Geometry: final body of the model. Coordinates: model frame, mm. Face numbers are marked on the shaded views. A direction names the side the tool comes from. Coordinates: 2 decimals unless noted, no trailing zeros. Order: outer loops, then holes, each group sorted by start corner. A loop starts at its lowest first (then second) coordinate and runs counter-clockwise, first axis right, second up. Notation, with made-up numbers: M 8,9.5 L 42,9.5 A8 cw 42,16.5 Z; hole C 70,74.5 d1. An arc over 180 degrees is marked long. Use CSV: the item, a comma, the result in double quotes. Start each with the question number.
1. Section query D-D on x = 40. Return the cut outline in (y, z), and give its area (3 significant figures).
2. Set-up query: the marked faces 4 and 5. Return all of +Z, -Z, +X, -X, +Y, -Y with unobstructed straight access to the full face (end or side cutting, diameter ignored); none if empty.
3. Pull-direction query (Y, two-part tool) for the marked faces 1, 2 and 3; classes: pulls with the +Y half, pulls with the -Y half, needs draft (parallel to the pull), parting line crosses it, or undercut.
4. First-contact query: P1, Ø4.5, axis at x = -15.5, y = -15.5, coming from the -Z side; P2, Ø2, axis at x = -17, y = 11, coming from the +Z side; P3, Ø12, axis at x = -18, z = 2.5, coming from the -Y side. Flat tips, straight axial feed; report the tip coordinate or a pass-through.
5. Section query A-A on y = 0. Return the cut outline in (x, z).
6. Section query B-B on z = 8.5. Return the cut outline in (x, y), and give its area (3 significant figures).
7. Material intervals for line 1 (Y direction, x = -15.5, z = 2.9); line 2 (Y direction, x = -15.5, z = 9.75), sorted ascending.
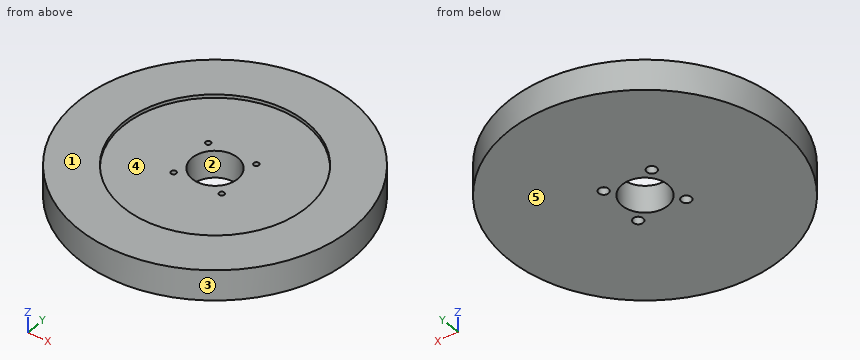
Autodesk Fusion 360 part; units mm, degrees
sketch "Sketch1" plane through (0, 0, 0) normal (0, 0, 1) x (1, 0, 0)
  circle A0 centre (0, 0) radius 90
  circle A1 centre (0, 0) radius 15
  line L0 (15.5, 15.5) -> (-15.5, 15.5)
  line L1 (-15.5, 15.5) -> (-15.5, -15.5)
  line L2 (-15.5, -15.5) -> (15.5, -15.5)
  line L3 (15.5, -15.5) -> (15.5, 15.5)
  line L4 (15.5, 15.5) -> (-15.5, -15.5) construction
  line L5 (-15.5, 15.5) -> (15.5, -15.5) construction
  circle A2 centre (-15.5, 15.5) radius 1.7
  circle A3 centre (15.5, 15.5) radius 1.7
  circle A4 centre (-15.5, -15.5) radius 1.7
  circle A5 centre (15.5, -15.5) radius 1.7
  dimension "d1" = 180
  dimension "d2" = 30
  dimension "d3" = 31
  dimension "d4" = 31
  dimension "d5" = 3.4
  dimension "d8" = 31
  dimension "d9" = -31
extrude "Extrude1" add sketch "Sketch1" along normal blind 20 contours A0 | L0 L1 L2 L3 A2 A3 A4 A5
sketch "Sketch2" plane through (0, 0, 20) normal (0, 0, 1) x (-1, 0, 0)
  circle A0 centre (0, 0) radius 15
  circle A1 centre (15.5, -15.5) radius 1.7
  circle A2 centre (15.5, 15.5) radius 1.7
  circle A3 centre (-15.5, -15.5) radius 1.7
  circle A4 centre (-15.5, 15.5) radius 1.7
  circle A5 centre (0, 0) radius 90
  circle A6 centre (0, 0) radius 60.25
  dimension "d12" = 120.5
extrude "Extrude2" cut sketch "Sketch2" against normal blind 2.2 contours A6
hole "Hole1" at (15.5, -15.5, 0) direction (0, 0, 1) diameter 3.2 depth 17.8 tip angle 118 counterbore diameter 6.5 counterbore depth 5
hole "Hole2" at (15.5, 15.5, 0) direction (0, 0, 1) diameter 3.2 depth 17.8 tip angle 118 counterbore diameter 6.5 counterbore depth 5
hole "Hole3" at (-15.5, -15.5, 0) direction (0, 0, 1) diameter 3.2 depth 17.8 tip angle 118 counterbore diameter 6.5 counterbore depth 5
hole "Hole4" at (-15.5, 15.5, 0) direction (0, 0, 1) diameter 3.2 depth 17.8 tip angle 118 counterbore diameter 6.5 counterbore depth 5
Results list:
1,outline,"M -80.62,0 L 80.62,0 L 80.62,20 L 45.06,20 L 45.06,17.8 L -45.06,17.8 L -45.06,20 L -80.62,20 Z"
1,area,"3,030 mm²"
2,face 4,"+Z"
2,face 5,"-Z, +X, -X, +Y, -Y"
3,face 1,"needs draft"
3,face 2,"undercut"
3,face 3,"parting line crosses it"
4,P1,"stops at z = 5"
4,P2,"stops at z = 17.8"
4,P3,"stops at y = -89.2"
5,outline,"M -90,0 L -15,0 L -15,17.8 L -60.25,17.8 L -60.25,20 L -90,20 Z; M 15,0 L 90,0 L 90,20 L 60.25,20 L 60.25,17.8 L 15,17.8 Z"
6,outline,"C 0,0 d180; hole C -15.5,-15.5 d3.4; hole C -15.5,15.5 d3.4; hole C 0,0 d30; hole C 15.5,-15.5 d3.4; hole C 15.5,15.5 d3.4"
6,area,"24,700 mm²"
7,line 1,"y = -88.66 to -18.75, -12.25 to 12.25, 18.75 to 88.66"
7,line 2,"y = -88.66 to -17.2, -13.8 to 13.8, 17.2 to 88.66"
